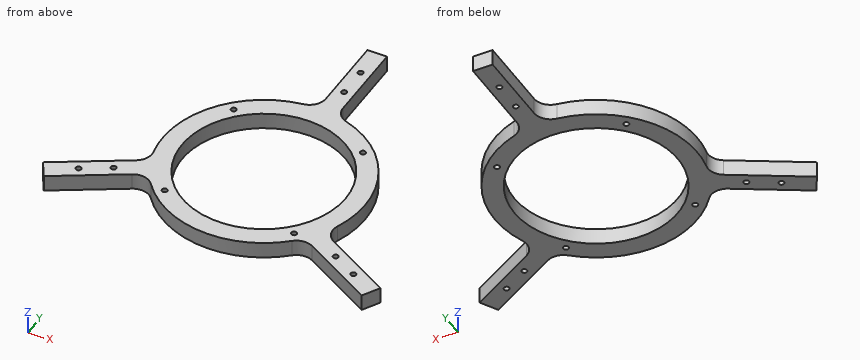
from build123d import *

# Parameters (mm, degrees)
SKETCH_1_R             = 50
EXTRUDE_1_DEPTH        = 10
HOLE_WIZARD_M4_1_D     = 3.3
HOLE_WIZARD_M4_1_DEPTH = 10.1
HOLE_WIZARD_M4_1_TIP   = 0.991420021
FILLET_1_R             = 10


with BuildPart() as part:
    # 草图1 → 凸台-拉伸1 (new body)
    with BuildSketch(Plane.XY):
        with BuildLine():
            Line((12, 60.827625303), (12, 119))
            Line((12, 119), (0, 119))
            Line((0, 119), (0, 62))
            ThreePointArc((0, 62), (-50.42486234, 36.073996979), (-58.678268764, -20.021507806))
            Line((-58.678268764, -20.021507806), (-109.05702305, -49.107695155))
            Line((-109.05702305, -49.107695155), (-103.05702305, -59.5))
            Line((-103.05702305, -59.5), (-53.693575035, -31))
            ThreePointArc((-53.693575035, -31), (-6.02856663, -61.706210258), (46.678268764, -40.806117497))
            Line((46.678268764, -40.806117497), (97.05702305, -69.892304845))
            Line((97.05702305, -69.892304845), (103.05702305, -59.5))
            Line((103.05702305, -59.5), (53.693575035, -31))
            ThreePointArc((53.693575035, -31), (56.453428969, 25.632213279), (12, 60.827625303))
        make_face()
        Circle(SKETCH_1_R, mode=Mode.SUBTRACT)
    extrude(amount=EXTRUDE_1_DEPTH)

    # M4 螺纹孔1
    with Locations(Plane.XY.offset(10)):
        with Locations((-39.597979746, 39.597979746), (-39.597979746, -39.597979746), (39.597979746, -39.597979746), (39.597979746, 39.597979746), (-89.602540378, -44.803847577), (-73.148057707, -35.303847577), (84.468565782, -55.696152423), (68.880108514, -46.696152423), (6, 81), (6, 100)):
            Hole(HOLE_WIZARD_M4_1_D / 2, depth=HOLE_WIZARD_M4_1_DEPTH)
            with Locations((0, 0, -(HOLE_WIZARD_M4_1_DEPTH + HOLE_WIZARD_M4_1_TIP / 2))):  # 118° drill point
                Cone(0, HOLE_WIZARD_M4_1_D / 2, HOLE_WIZARD_M4_1_TIP, mode=Mode.SUBTRACT)

    # 圆角1
    fillet_1_edges = [part.edges().sort_by_distance(p)[0] for p in [
        (-58.678268764, -20.021507806, 5),
        (0, 62, 5),
        (12, 60.827625303, 5),
        (53.693575035, -31, 5),
        (46.678268764, -40.806117497, 5),
        (-53.693575035, -31, 5),
    ]]
    fillet(fillet_1_edges, radius=FILLET_1_R)


solid = part.part
Input: part model. Units: mm. Frame: model coordinates. Give positions to 0.01 mm unless a question says otherwise; leave off trailing zeros. Loops run counter-clockwise (first coordinate to the right, second up) from the corner with the lowest first, then second, coordinate; pieces in that order, holes last. Notation, with made-up numbers: (33.25, -14.75) -> (47.25, -14.75) arc R15 cw to (47.25, 7.25) -> close; hole circle Ø2 at (47, -37.5). An arc over 180 degrees is marked (long way). Answer as a JSON object with one key per item and string values. Group by question number.
Item 1: Line query: probe 1 along X at (y, z) = (40.5, 5.75); probe 2 along X at (y, z) = (100, 5.25); probe 3 along Y at (x, z) = (6, 4.5). Output: solid intervals per line, ascending.
Item 2: Cut plane C-C, the plane y = -20. Return the cut outline in (x, z) (3 decimals), and give its area (3 significant figures).
Item 3: Pin query (flat end, axial travel): P1, Ø4, axis at x = 39.6, y = -39.6, coming from the +Z side; P2, Ø1.5, axis at y = -12, z = 4, coming from the +X side; P3, Ø1, axis at y = -6.5, z = 2, coming from the +X side; P4, Ø3, axis at y = -32, z = 8.5, coming from the -X side. Return the tip coordinate at first contact, or that it passes through.
Item 4: Cut plane A-A, the plane y = 0. Return the cut outline in (x, z).
Item 5: Cut plane B-B, the plane z = 7.25. State how many separate pieces and enclosed holes the cut face has, and give its area (3 significant figures).
Item 6: Cut plane D-D, the plane x = 75. Return the cut outline in (y, z), and give its area (3 significant figures).
Checks:
{
 "1": {"probe 1": "x = -46.94 to -40.98, -38.22 to -29.32, 29.32 to 38.22, 40.98 to 46.94", "probe 2": "x = 0 to 4.35, 7.65 to 12", "probe 3": "y = -61.71 to -49.64, 49.64 to 79.35, 82.65 to 98.35, 101.65 to 119"},
 "2": {"outline": "(-61.585, 0) -> (-45.826, 0) -> (-45.826, 10) -> (-61.585, 10) -> close; (45.826, 0) -> (58.686, 0) -> (58.686, 10) -> (45.826, 10) -> close", "area": "286 mm²"},
 "3": {"P1": "stops at z = 10", "P2": "stops at x = 60.97", "P3": "stops at x = 61.71", "P4": "stops at x = -82.02"},
 "4": {"outline": "(-62, 0) -> (-50, 0) -> (-50, 10) -> (-62, 10) -> close; (50, 0) -> (62, 0) -> (62, 10) -> (50, 10) -> close"},
 "5": {"separate pieces": "1", "enclosed holes": "11", "area": "6,290 mm²"},
 "6": {"outline": "(-57.16, 0) -> (-43.3, 0) -> (-43.3, 10) -> (-57.16, 10) -> close", "area": "139 mm²"}
}
